Check sheet for the modelled part. Datum: model origin and axes. Units: mm. Face numbers are marked on the shaded views. A direction names the side the tool comes from. Round coordinates to 2 decimals unless told otherwise and drop trailing zeros. Write each loop counter-clockwise with the first axis right and the second up, starting at its lowest first coordinate (ties: lowest second). Pieces come first, ordered by that corner, then holes.
Item 1: Material ranges on line 1 along Z through (x, y) = (10, 4.5); line 2 along X through (y, z) = (4, 0); line 3 along Y through (x, z) = (67, 0), recorded low to high.
Item 2: Set-up check for the marked faces 1 and 2: record each of +Z, -Z, +X, -X, +Y, -Y from which the full face is reachable in a straight line by a thin tool's end or side.
Item 3: Section check D-D, the plane x = 22. Record the cut outline in (y, z), plus the area to 3 significant figures.
Item 4: Depth check by flat-ended pin: pin 1 (5 mm diameter, centred on y = 50, z = -1.5, fed in from -X); pin 2 (7 mm diameter, centred on y = 88.5, z = 1, fed in from -X); pin 3 (8 mm diameter, centred on y = 87, z = 0, fed in from -X). Enter the tip coordinate at first touch or a pass-through.
Item 5: Section check C-C, the plane x = 48.5. Record the cut outline in (y, z).
Item 6: Section check B-B, the plane x = 10. Record the cut outline in (y, z), plus the area to 3 significant figures.
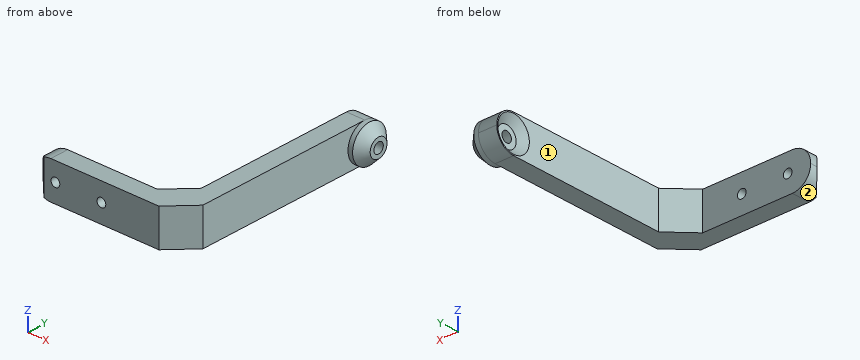
Autodesk Inventor part; units mm, degrees
ref_plane "YZ Plane" through (0, 0, 0) normal (1, 0, 0) x (0, 1, 0)
ref_plane "XZ Plane" through (0, 0, 0) normal (0, 1, 0) x (-1, 0, 0)
ref_plane "XY Plane" through (0, 0, 0) normal (0, 0, 1) x (1, 0, 0)
sketch "Sketch3" plane through (0, 0, 0) normal (0, 0, 1) x (1, 0, 0)
  line L0 (0, 0) -> (65, 0)
  line L1 (65, 0) -> (65, 95)
  line L2 (65, 95) -> (57, 95)
  line L3 (57, 95) -> (57, 8)
  line L4 (57, 8) -> (0, 8)
  line L5 (0, 8) -> (0, 0)
  dimension "d17" = 8
  dimension "d18" = 57
  dimension "d19" = 87
  dimension "d20" = 8
extrude "Extrusion3" add sketch "Sketch3" against normal mid plane 16
sketch "Sketch5" plane through (0, 8, -8) normal (0, 1, 0) x (1, 0, 0)
  line L0 (-13, -8) -> (78, -8)
  circle A0 centre (10, -8) radius 1.9
  circle A1 centre (30, -8) radius 1.9
  line L1 (0, 0) -> (0, -16)
  point P0 (0, -8)
  dimension "d23" = 3.8
  dimension "d24" = 3.8
  dimension "d25" = 10
  dimension "d26" = 20
extrude "Extrusion4" cut sketch "Sketch5" against normal through all
chamfer "Chamfer2" distance 5 angle 45 1 edges at (0, 0, 0)
chamfer "Chamfer3" distance 10 angle 45 1 edges at (57, 8, 0)
chamfer "Chamfer4" distance 10 angle 45 1 edges at (65, 0, 0)
sketch "Sketch6" plane through (65, 95, 8) normal (1, 0, 0) x (0, 0, -1)
  line L0 (16, -77) -> (16, 0)
  line L1 (0, -85) -> (0, 0)
  circle A0 centre (8, -8) radius 8
  line L2 (16, 0) -> (0, 0)
  point P0 (8, -95)
  dimension "d39" = 16
extrude "Extrusion5" add sketch "Sketch6" along normal blind 7 contours A0
fillet "Fillet1" radius 8 2 edges at (61, 95, -8) (61, 95, 8)
sketch "Sketch7" plane through (57, 18, -8) normal (-1, 0, 0) x (0, 0, 1)
  point P0 (8, -18)
sketch "Sketch8" plane through (72, 87, 0) normal (1, 0, 0) x (0, 0, -1)
  circle A0 centre (0, 0) radius 8
  circle A1 centre (0, 0) radius 2.75
  point P0 (0, -87)
  dimension "d43" = 5.5
extrude "Extrusion6" add sketch "Sketch8" along normal blind 4 contours A1
sketch "Sketch9" plane through (76, 87, 0) normal (1, 0, 0) x (0, 0, -1)
  circle A0 centre (0, 0) radius 2.75 construction
  circle A1 centre (0, 0) radius 2.25
  point P0 (0, -87)
  dimension "d46" = 4.5
extrude "Extrusion7" cut sketch "Sketch9" against normal through all
sketch "Sketch10" plane through (57, 18, -8) normal (-1, 0, 0) x (0, 0, 1)
  circle A0 centre (8, 69) radius 2.25
  circle A1 centre (8, 69) radius 4.5
  point P0 (8, -18)
  dimension "d49" = 9
extrude "Extrusion8" cut sketch "Sketch10" against normal blind 3
chamfer "Chamfer5" distance 3 angle 45 1 edges at (57, 87, -4.5)
chamfer "Chamfer6" distance 3 angle 45 1 edges at (72, 87, 2.75)
fillet "Fillet2" radius 8 2 edges at (0, 6.5, -8) (0, 6.5, 8)
sketch "Sketch11" plane through (76, 87, 0) normal (1, 0, 0) x (0, 0, -1)
  circle A0 centre (0, 0) radius 2.25
  circle A1 centre (0, 0) radius 2.75
  circle A2 centre (0, 0) radius 10.0452
  point P0 (0, -87)
extrude "Extrusion9" cut sketch "Sketch11" against normal blind 5 contours A0 | A1 | A2
chamfer "Chamfer7" distance 4 angle 45 1 edges at (71, 87, 8)
equation "\"d20\" = d17"
properties part number "_3DPrint"
Values found:
1. line 1: z = -8 to -1.9, 1.9 to 8
1. line 2: x = 1 to 8.1, 11.9 to 28.1, 31.9 to 59
1. line 3: y = 79 to 84.75, 89.25 to 95
2. face 1: +Z, -Z, -X, +Y
2. face 2: -Z, -X, +Y, -Y
3. outline: (0, -8) - (8, -8) - (8, 8) - (0, 8) - close
3. area: 128 mm2
4. pin 1: stops at x = 57
4. pin 2: stops at x = 59.2
4. pin 3: stops at x = 60
5. outline: (0, -8) - (9.5, -8) - (9.5, 8) - (0, 8) - close
6. outline: (0, -8) - (8, -8) - (8, -1.9) - (0, -1.9) - close; (0, 1.9) - (8, 1.9) - (8, 8) - (0, 8) - close
6. area: 97.6 mm2
